from build123d import *

# Parameters (mm, degrees)
SKETCH032_R  = 1.75
PAD005_DEPTH = 5
CHAMFER_SIZE = 1.4
FILLET002_R  = 4.4


with BuildPart() as part:
    # Sketch032 → Pad005 (new body)
    with BuildSketch(Plane.XZ):
        with BuildLine():
            Line((-30, 17), (30, 17))
            ThreePointArc((36, 11), (34.242641, 15.242641), (30, 17))
            Line((36, 11), (36, -22))
            ThreePointArc((34, -24), (35.414214, -23.414214), (36, -22))
            Line((34, -24), (-34, -24))
            ThreePointArc((-36, -22), (-35.414214, -23.414214), (-34, -24))
            Line((-36, -22), (-36, 11))
            ThreePointArc((-30, 17), (-34.242641, 15.242641), (-36, 11))
        make_face()
        with Locations((-29, 8.9)):
            Circle(SKETCH032_R, mode=Mode.SUBTRACT)
        with Locations((0, 8.9)):
            Circle(SKETCH032_R, mode=Mode.SUBTRACT)
        with Locations((29, 8.9)):
            Circle(SKETCH032_R, mode=Mode.SUBTRACT)
        with Locations((-27.5, -16.6)):
            Circle(SKETCH032_R, mode=Mode.SUBTRACT)
        with Locations((27.5, -16.6)):
            Circle(SKETCH032_R, mode=Mode.SUBTRACT)
    extrude(amount=PAD005_DEPTH)

    # Chamfer
    chamfer_edges = [part.edges().sort_by_distance(p)[0] for p in [
        (25.75, 0, -16.6),
        (-30.75, 0, 8.9),
        (-1.75, 0, 8.9),
        (27.25, 0, 8.9),
        (-29.25, 0, -16.6),
    ]]
    chamfer(chamfer_edges, length=CHAMFER_SIZE)

    # Fillet002
    fillet002_edges = [part.edges().sort_by_distance(p)[0] for p in [
        (36, 0, -5.5),
        (34.242641, 0, 15.242641),
        (0, 0, 17),
        (-34.242641, 0, 15.242641),
        (-36, 0, -5.5),
        (-35.414214, 0, -23.414214),
        (0, 0, -24),
        (35.414214, 0, -23.414214),
    ]]
    fillet(fillet002_edges, radius=FILLET002_R)


with BuildPart() as part_1:
    # Body placement: moved
    add(part.part.moved(Location((0, 46, 0))))


solid = part_1.part
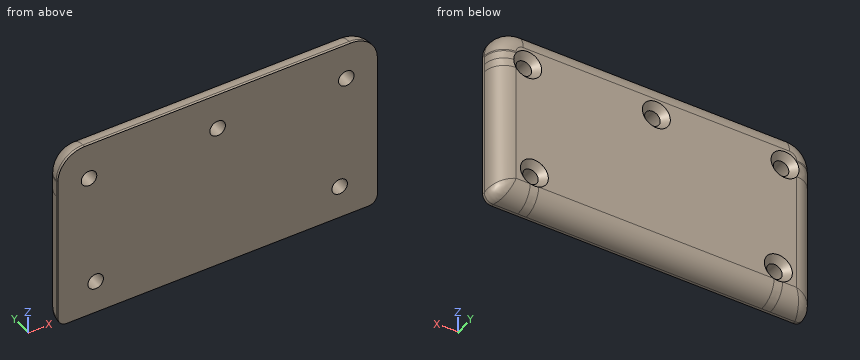
Could you check a few things on this model? Use its own coordinates, in mm. Give positions to 0.01 mm unless a question says otherwise; leave off trailing zeros. Order: outer loops, then holes, each group sorted by start corner. A loop starts at its lowest first (then second) coordinate and runs counter-clockwise, first axis right, second up. Notation, with made-up numbers: M 46,-29 L 99,-29 A37 ccw 99,7 Z; hole C 37,10.5 d6. An arc over 180 degrees is marked long. One line per question, with ' | ' between items.
1. I want a section at A-A (x = 0). List the corners of the cut face in (y, z) for me.
Results:
outline: M 41,-24 L 41.6,-24 A4.4 ccw 46,-19.6 L 46,5.75 L 44.6,7.15 L 41,7.15 Z; M 41,10.65 L 44.6,10.65 L 46,12.05 L 46,12.6 A4.4 ccw 41.6,17 L 41,17 Z
2. If I drill on line 1 (X direction, y = 42.95, z = -16.5); line 2 (X direction, y = 45.2, z = -17.5); line 3 (Z direction, x = 29, y = 42.2), over which ranges is the centre line in solid material (lowest first)?
Results:
line 1: -35.79 to -29.25, -25.75 to 25.75, 29.25 to 35.79 | line 2: -34.13 to -29.67, -25.33 to 25.33, 29.67 to 34.13 | line 3: -23.96 to -17.5, -15.7 to 7.15, 10.65 to 16.96
3. I want a section at B-B (x = -12). List the corners of the cut face in (y, z) for me.
Results:
outline: M 41,-24 L 41.6,-24 A4.4 ccw 46,-19.6 L 46,12.6 A4.4 ccw 41.6,17 L 41,17 Z
4. I want a section at C-C (y = 42.35). Give the number of separate pieces and of enclosed holes in the cut face, and give its area (3 significant figures).
Results:
separate pieces: 1 | enclosed holes: 5 | area: 2,870 mm²
5. I'm going to push flat-ended pins straight in: pin 1 (4 mm diameter, centred on x = 0, z = 8.9, fed in from +Y); pin 2 (1 mm diameter, centred on y = 44.5, z = -3.5, fed in from -X); pin 3 (3 mm diameter, centred on y = 45.5, z = 11.5, fed in from +X). Where does each tip first touch, or does it pass through?
Results:
pin 1: y = 44.85 | pin 2: x = -35.29 | pin 3: x = 35.27
